from build123d import *

# Parameters (mm, degrees)
COVER_START          = -375.38
COVER_DEPTH          = 439.28
RAIL_START           = -378.38
RAIL_FLANGE_DEPTH    = 445.28
SKETCH3_R            = 22
OIL_FILLER_CAP_DEPTH = 16


with BuildPart() as part:
    # Sketch1 → Cover (new body)
    with BuildSketch(Plane.XY.offset(COVER_START)):
        with BuildLine():
            Line((193.711902706, 287.049997823), (287.049997823, 193.711902706))
            Line((287.049997823, 193.711902706), (305.717616846, 212.379521729))
            ThreePointArc((305.717616846, 212.379521729), (312.044110372, 227.653028203), (305.717616846, 242.926534677))
            Line((305.717616846, 242.926534677), (242.926534677, 305.717616846))
            ThreePointArc((242.926534677, 305.717616846), (227.653028203, 312.044110372), (212.379521729, 305.717616846))
            Line((212.379521729, 305.717616846), (193.711902706, 287.049997823))
        make_face()
    extrude(amount=COVER_DEPTH)

    # Sketch2 → Rail Flange (add)
    with BuildSketch(Plane.XY.offset(RAIL_START)):
        Polygon((191.590582362, 289.171318166), (289.171318166, 191.590582362), (293.413958853, 195.83322305), (195.83322305, 293.413958853), align=None)
    extrude(amount=RAIL_FLANGE_DEPTH)

    # Sketch3 → Oil Filler Cap (add)
    with BuildSketch(Plane(origin=(274.322075761, 274.322075761, 0), x_dir=(0, 0, -1), z_dir=(0.7071067811865477, 0.7071067811865475, 0))):
        with Locations(Location((34, 0, 0), (0, 0, 270))):
            Circle(SKETCH3_R)
    extrude(amount=OIL_FILLER_CAP_DEPTH)


solid = part.part
CAD build for the part. Positions are in the model's coordinates, mm. A direction names the side the tool comes from. Give positions to 0.01 mm unless a question says otherwise; leave off trailing zeros. Write each loop counter-clockwise with the first axis right and the second up, starting at its lowest first coordinate (ties: lowest second). Pieces come first, ordered by that corner, then holes. Notation, with made-up numbers: (50, 27) - (103, 27) arc R28 ccw to (103, 53) - close; hole circle Ø3 at (-32, 63). An arc over 180 degrees is marked (long way). Answer as CSV lines item,"result".
Q1. Flat gauge pins, fed straight in: pin 1 Ø6 at (y, z) = (215.5, -133.5) entering from +X; pin 2 Ø2 at (x, y) = (246, 275) entering from +Z; pin 3 Ø4 at (x, z) = (267.5, -135) entering from +Y. Where does each tip first touch, or does it go through?
Result set:
pin 1,"x = 310.01"
pin 2,"z = 63.9"
pin 3,"y = 283.14"
Q2. Band-saw the part on C-C (x = 208.5). Give the cut face in (y, z).
Result set:
outline,"(272.26, -378.38) - (280.75, -378.38) - (280.75, -375.38) - (301.84, -375.38) - (301.84, 63.9) - (280.75, 63.9) - (280.75, 66.9) - (272.26, 66.9) - close"
Q3. Band-saw the part on A-A (z = -217.5). Give the cut face in (x, y), and give its area (3 significant figures).
Result set:
outline,"(191.59, 289.17) - (289.17, 191.59) - (293.41, 195.83) - (291.29, 197.95) - (305.72, 212.38) arc R21.6 ccw to (305.72, 242.93) - (242.93, 305.72) arc R21.6 ccw to (212.38, 305.72) - (197.95, 291.29) - (195.83, 293.41) - close"
area,"6,170 mm²"
Q4. Drill centre lines: line 1 (Y direction, x = 291.5, z = -45.5); line 2 (Z direction, x = 268, y = 260); line 3 (X direction, y = 263, z = -346). Where is each one in solid material? Low to high. Write a range as from..to.
Result set:
line 1,"193.92..197.75, 198.16..257.14, 264.98..279.77"
line 2,"-375.38..63.9"
line 3,"217.76..285.64"
Q5. Pull direction X, two halves, no side cores. Call faces 1 (the face through (254, 256, 63.9)), 2 (the face through (291.835, 197.413, -156.779)), 3 (the face through (239.7, 241.06, -158.86)): released by +X, released by -X, zero draft, split by the parting line, or undercut.
Result set:
face 1,"zero draft"
face 2,"undercut"
face 3,"released by -X"
Q6. 3-axis set-ups, long thin cutter, end or side, ignore diameter. For faces 4 (the face through (254, 256, -375.38)), 5 (the face through (287.1, 272.7, -14.5)): which of +Z, -Z, +X, -X, +Y, -Y reach the whole face in a straight line?
Result set:
face 4,"-Z, +X, +Y"
face 5,"none"
Q7. Band-saw the part on B-B (y = 253.5). Give the cut face in (x, z), and give its area (3 significant figures).
Result set:
outline,"(227.26, -378.38) - (235.75, -378.38) - (235.75, -375.38) - (295.14, -375.38) - (295.14, 63.9) - (235.75, 63.9) - (235.75, 66.9) - (227.26, 66.9) - close"
area,"29,900 mm²"
